Source: CAD feature listing. Evaluate the final solid. Frame: model axes, mm. A direction names the side the tool comes from. Coordinates: 2 decimals unless noted, no trailing zeros. Loops run counter-clockwise (first coordinate to the right, second up) from the corner with the lowest first, then second, coordinate; pieces in that order, holes last.
Item 1: Pin query (flat end, axial travel): pin 1 Ø2.5 at (y, z) = (0.5, 2) entering from -X; pin 2 Ø1 at (y, z) = (-2, 17) entering from +X; pin 3 Ø3 at (x, z) = (1.5, 9.5) entering from -Y; pin 4 Ø2.5 at (x, z) = (-0.5, 1) entering from +Y. Return the tip coordinate at first contact, or that it passes through.
Item 2: Section query A-A, the plane x = 0. Return the cut outline in (y, z), then the cut area to 3 significant figures.
Item 3: Section query C-C, the plane z = 21.5. Return the cut outline in (x, y).
Item 4: Pull-direction query (Y, two-part tool) for faces 4 (the cylindrical face through (-0.29, 2.23, 1.73)), 5 (the flat face through (0, 0, 25)), 6 (the flat face through (0, -1.2, 1)); classes: +Y half, -Y half, draft (parallel to the pull), parting line (faces both ways), or undercut.
Item 5: Line query: probe 1 along X at (y, z) = (-0.2, 18.25); probe 2 along Y at (x, z) = (-0.15, 21). Output: solid intervals per line, ascending.
Item 6: Reachability of faces 1 (the cylindrical face through (0, 1, 12)), 2 (the flat face through (1.2, 0, 1)), 3 (the cylindrical face through (-3, 0, 22)) from +Z, -Z, +X, -X, +Y, -Y: full face, straight path, thin tool, end or side. Return the list, or none.
Item 7: Section query D-D, the plane z = 11.5. Return the cut outline in (x, y), then the cut area to 3 significant figures.
```python
from build123d import *

# Parameters (mm, degrees)
SKETCH_1_R          = 2.25
EXTRUDE_2_DEPTH     = 20
SKETCH_7_W          = 2.4
SKETCH_7_H          = 2.4
CUT_EXTRUDE_3_DEPTH = 2.5
SKETCH_9_R          = 3
EXTRUDE_4_DEPTH     = 5
CUT_EXTRUDE_START   = -20
SKETCH_12_OUTSIDE_W = 13.28
SKETCH_12_OUTSIDE_H = 13.28
SKETCH_12_OUTSIDE_R = 1
CUT_EXTRUDE_4_DEPTH = 16.5
FILLET_2_R          = 2
FILLET_3_R          = 0.5


with BuildPart() as part:
    # 草图1 → 凸台-拉伸2 (new body)
    with BuildSketch(Plane.XY):
        Circle(SKETCH_1_R)
    extrude(amount=EXTRUDE_2_DEPTH)

    # 草图7 → 切除-拉伸3 (cut)
    with BuildSketch(Plane.XY):
        Rectangle(SKETCH_7_W, SKETCH_7_H)
    extrude(amount=CUT_EXTRUDE_3_DEPTH, mode=Mode.SUBTRACT)

    # 草图9 → 凸台-拉伸4 (add)
    with BuildSketch(Plane.XY.offset(20)):
        Circle(SKETCH_9_R)
    extrude(amount=EXTRUDE_4_DEPTH)

    # 草图12 outside → 切除-拉伸4 (cut)
    with BuildSketch(Plane(origin=(0, 0, 0), x_dir=(-1, 0, 0), z_dir=(0, 0, -1)).offset(CUT_EXTRUDE_START)):
        Rectangle(SKETCH_12_OUTSIDE_W, SKETCH_12_OUTSIDE_H)
        with Locations(Location((0, 0, 0), (0, 0, 180))):
            Circle(SKETCH_12_OUTSIDE_R, mode=Mode.SUBTRACT)
    extrude(amount=CUT_EXTRUDE_4_DEPTH, mode=Mode.SUBTRACT)

    # 圆角2
    # the kernel refuses this fillet: 2 mm, written as the material it adds along each edge
    with BuildSketch(Plane(origin=(0, 0, 3.5), x_dir=(1, 0, 0), z_dir=(0, 1, 0))) as fillet_2_piece_1:
        with BuildLine():
            CenterArc((3, -1.854049622), FILLET_2_R, 112.024312837, 67.975687163)
            Line((2.25, 0), (2.235, 0.037080992))
            ThreePointArc((2.235, 0.037080992), (1.625, 0.04), (1, 0.04))
            Line((1, 0.04), (0.96, 0))
            Line((0.96, 0), (0.96, -1.854049622))
            Line((0.96, -1.854049622), (1, -1.854049622))
        make_face()
    revolve(axis=Axis((0, 0, 3.5), (0, 0, -1)))
    with BuildSketch(Plane(origin=(0, 0, 20), x_dir=(1, 0, 0), z_dir=(0, 1, 0))) as fillet_2_piece_2:
        with BuildLine():
            CenterArc((1 + FILLET_2_R, FILLET_2_R), FILLET_2_R, 180, 90)
            Line((1, FILLET_2_R), (1 - FILLET_2_R * 0.02, FILLET_2_R))
            Line((1 - FILLET_2_R * 0.02, FILLET_2_R), (1 - FILLET_2_R * 0.02, -FILLET_2_R * 0.02))
            Line((1 - FILLET_2_R * 0.02, -FILLET_2_R * 0.02), (1 + FILLET_2_R, -FILLET_2_R * 0.02))
            Line((1 + FILLET_2_R, -FILLET_2_R * 0.02), (1 + FILLET_2_R, 0))
        make_face()
    revolve(axis=Axis((0, 0, 20), (0, 0, -1)))

    # 圆角3
    fillet_3_edges = [part.edges().sort_by_distance(p)[0] for p in [
        (-3, 0, 25),
    ]]
    fillet(fillet_3_edges, radius=FILLET_3_R)


solid = part.part
```
Verdict:
1. pin 1: stops at x = -2.25
1. pin 2: passes through
1. pin 3: stops at y = -1
1. pin 4: stops at y = 2.25
2. outline: (-3, 20) arc R2 cw to (-1, 18) - (-1, 5.35) arc R2 cw to (-2.25, 3.5) - (-2.25, 0) - (-1.2, 0) - (-1.2, 2.5) - (1.2, 2.5) - (1.2, 0) - (2.25, 0) - (2.25, 3.5) arc R2 cw to (1, 5.35) - (1, 18) arc R2 cw to (3, 20) - (3, 24.5) arc R0.5 ccw to (2.5, 25) - (-2.5, 25) arc R0.5 ccw to (-3, 24.5) - close
2. area: 75.6 mm2
3. outline: circle Ø6 at (0, 0)
4. face 4: parting line
4. face 5: draft
4. face 6: undercut
5. probe 1: x = -1 to 1
5. probe 2: y = -3 to 3
6. face 1: none
6. face 2: -Z
6. face 3: +Z, -Z
7. outline: circle Ø2 at (0, 0)
7. area: 3.14 mm2
